Could you check a few things on this model? Use its own coordinates, in mm. Face numbers are marked on the shaded views. A direction names the side the tool comes from. Give positions to 0.01 mm unless a question says otherwise; leave off trailing zeros. Order: outer loops, then holes, each group sorted by start corner. A loop starts at its lowest first (then second) coordinate and runs counter-clockwise, first axis right, second up. Notation, with made-up numbers: M 14.25,75 L 65.25,75 A15 ccw 65.25,80 Z; hole C -37,50 d4. An arc over 180 degrees is marked long. Use a Markdown table: item, result. Add a question column.
Autodesk Inventor part; units mm, degrees
ref_plane "YZ Plane" through (0, 0, 0) normal (1, 0, 0) x (0, 1, 0)
ref_plane "XZ Plane" through (0, 0, 0) normal (0, 1, 0) x (-1, 0, 0)
ref_plane "XY Plane" through (0, 0, 0) normal (0, 0, 1) x (1, 0, 0)
sketch "Sketch1" plane through (0, 0, 0) normal (0, 1, 0) x (-1, 0, 0)
  line L0 (0, 0) -> (-12.7, 0)
  line L1 (-12.7, 0) -> (-12.7, -1.5875)
  line L2 (-12.7, -1.5875) -> (0, -1.5875)
  line L3 (0, -1.5875) -> (0, 0)
  line L4 (0, 0) -> (-4.318, 0)
  line L5 (-4.318, 0) -> (-4.318, -12.7)
  line L6 (-4.318, -12.7) -> (0, -12.7)
  line L7 (0, -12.7) -> (0, 0)
  dimension "d0" = 4.318
  dimension "d1" = 12.7
  dimension "d2" = 12.7
  dimension "d33" = 1.5875
extrude "Extrusion1" add sketch "Sketch1" along normal blind 50.8
sketch "Sketch2" plane through (0, 50.8, 0) normal (0, 1, 0) x (1, 0, 0)
  line L0 (12.7, 0) -> (12.7, 1.5875)
  line L1 (12.7, 1.5875) -> (-4.064, 1.5875)
  line L2 (-4.064, 1.5875) -> (-4.064, -8.5725)
  line L3 (-4.064, -8.5725) -> (12.7, -8.5725)
  line L4 (12.7, -8.5725) -> (12.7, 1.5875)
  line L5 (4.318, 12.7) -> (-4.064, 12.7)
  line L6 (-4.064, 12.7) -> (-4.064, -8.5725)
  line L7 (-4.064, -8.5725) -> (4.318, -8.5725)
  line L8 (4.318, -8.5725) -> (4.318, 12.7)
  dimension "d26" = 10.16
  dimension "d28" = 16.764
extrude "Extrusion2" add sketch "Sketch2" along normal blind 6.35
sketch "Sketch5" plane through (0, 50.8, 0) normal (0, -1, 0) x (1, 0, 0)
  line L0 (12.7, 8.5725) -> (12.7, 0)
  line L1 (-4.064, -12.7) -> (-4.064, 8.5725)
  line L2 (12.7, 8.5725) -> (-4.064, 8.5725)
  line L3 (-4.064, 8.5725) -> (-4.064, 2.1082)
  line L4 (-4.064, 2.1082) -> (12.7, 2.1082)
  line L5 (12.7, 2.1082) -> (12.7, 8.5725)
  line L6 (0, -12.7) -> (-4.064, -12.7)
  line L7 (-4.064, 8.5725) -> (-2.1082, 8.5725)
  line L8 (-2.1082, 8.5725) -> (-2.1082, -12.7)
  line L9 (-2.1082, -12.7) -> (-4.064, -12.7)
  line L10 (-4.064, -12.7) -> (-4.064, 8.5725)
  line L11 (0, -12.7) -> (0, 0)
  line L12 (0, 0) -> (12.7, 0)
  dimension "d29" = 2.1082
  dimension "d30" = 2.1082
extrude "Extrusion4" add sketch "Sketch5" along normal blind 12.7 contours L0 L4 L8 L2 | L8 L4 L1 L2 | L8 L6 L1 L4
sketch "Sketch7" plane through (-4.064, 57.15, -12.7) normal (-1, 0, 0) x (0, 0, 1)
  line L0 (11.1125, 0) -> (11.1125, -57.15)
  line L1 (0, -57.15) -> (0, 0)
  line L2 (11.1125, 0) -> (0, 0)
  line L3 (0, -19.05) -> (14.8082, -19.05)
  line L4 (0, -6.35) -> (12.7, -6.35)
  point P0 (12.7, -57.15)
  point P1 (5.5562, -12.7)
  dimension "d47" = 11.1125
  dimension "d49" = 5.5563
  dimension "d58" = 12.7
  dimension "d59" = 6.35
hole "Hole2" at (-4.064, 44.45, -7.1438) direction (1, 0, 0) diameter 5.1562 depth 1.5875 tip angle 118
sketch "Sketch8" plane through (-4.064, 57.15, -12.7) normal (-1, 0, 0) x (0, 0, 1)
  circle A0 centre (5.5562, -12.7) radius 2.5781
  circle A1 centre (5.5562, -12.7) radius 2.5781
  line L0 (21.2725, 0) -> (21.2725, -19.05)
  line L1 (0, 0) -> (21.2725, 0)
  line L2 (0, -19.05) -> (0, 0)
  line L3 (21.2725, -19.05) -> (0, -19.05)
  point P0 (12.7, -57.15)
extrude "Extrusion5" add sketch "Sketch8" along normal blind 2.413
sketch "Sketch9" plane through (-2.1082, 50.8, 2.1082) normal (1, 0, 0) x (0, 0, -1)
  circle A0 centre (9.2519, -6.35) radius 2.5781
  line L0 (14.8082, -12.7) -> (-6.4643, -12.7)
  line L1 (6.6738, -6.35) -> (11.83, -6.35)
  line L2 (11.83, -6.35) -> (11.83, -12.7)
  line L3 (11.83, -12.7) -> (6.6738, -12.7)
  line L4 (6.6738, -12.7) -> (6.6738, -6.35)
  point P0 (2.1082, -50.8)
  dimension "d62" = 5.1562
extrude "Extrusion6" cut sketch "Sketch9" against normal blind 1.5875
equation "\"d29\" = d30"
properties part number "8GrootTelescope"
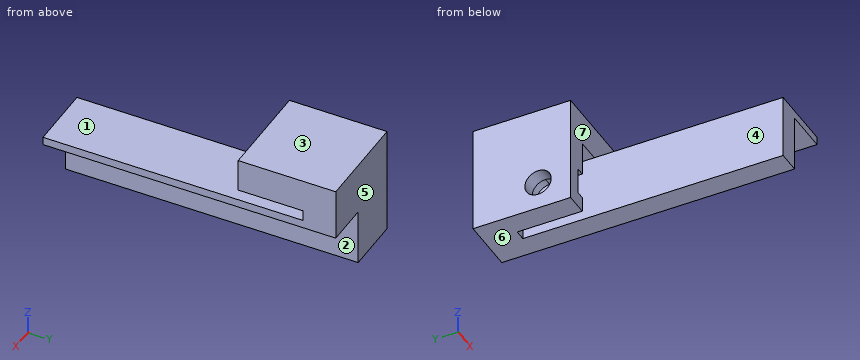
1) For the marked faces 1, 2, 3 and 4, which set-ups out of +Z, -Z, +X, -X, +Y, -Y let a thin tool reach every point of the face, with its end or its side?
2) We'd pull the mould along Y, two halves only. Please class the marked faces 5, 6 and 7: pulls with the +Y half, pulls with the -Y half, needs draft (parallel to the pull), parting line crosses it, or undercut.
3) Suppose I cut it at C-C on y = 37.5. Please give me the cut outline in (x, z).
4) Please list where these lines run through material, in increasing order: line 1 (Z direction, x = 5.75, y = 41); line 2 (Z direction, x = -3.55, y = 44.45); line 3 (Y direction, x = 10.25, z = 0.5). Write a range as from..to.
5) Suppose I cut it at B-B on z = -0.75. Please give me the cut outline in (x, y), and give its area (3 significant figures).
6) Suppose I cut it at A-A on x = 9.5. Please give me the cut outline in (y, z), and give its area (3 significant figures).
7) Suppose I cut it at D-D on z = 1.5. Please give me the cut outline in (x, y).
8) For pin 1 (1.5 mm diameter, centred on x = 5.5, y = 33, fed in from -Z); pin 2 (6.5 mm diameter, centred on y = 30.5, z = -5, fed in from -X); pin 3 (6 mm diameter, centred on y = 44.45, z = -7.14, fed in from +X), each with a flat end and sliding along its axis, tell me the tip position at first contact or that it passes through.
Values found:
| question | item | result |
|---|---|---|
| 1 | face 1 | +X, -Y |
| 1 | face 2 | -Z, +X, +Y, -Y |
| 1 | face 3 | +Z, +X, -X, +Y, -Y |
| 1 | face 4 | -Z, -Y |
| 2 | face 5 | pulls with the +Y half |
| 2 | face 6 | needs draft |
| 2 | face 7 | pulls with the -Y half |
| 3 | outline | M 0,-12.7 L 4.32,-12.7 L 4.32,-1.59 L 12.7,-1.59 L 12.7,0 L 0,0 Z |
| 4 | line 1 | z = -1.59..0, 2.11..8.57 |
| 4 | line 2 | z = -12.7..-9.72, -4.57..8.57 |
| 4 | line 3 | y = 50.8..57.15 |
| 5 | outline | M -6.48,38.1 L -2.11,38.1 L -2.11,50.8 L 0,50.8 L 0,0 L 12.7,0 L 12.7,57.15 L -6.48,57.15 Z |
| 5 | area | 822 mm^2 |
| 6 | outline | M 0,-1.59 L 57.15,-1.59 L 57.15,8.57 L 38.1,8.57 L 38.1,2.11 L 50.8,2.11 L 50.8,0 L 0,0 Z |
| 6 | area | 227 mm^2 |
| 7 | outline | M -6.48,38.1 L -2.11,38.1 L -2.11,50.8 L 12.7,50.8 L 12.7,57.15 L -6.48,57.15 Z |
| 8 | pin 1 | stops at z = -1.59 |
| 8 | pin 2 | stops at x = 0 |
| 8 | pin 3 | stops at x = 4.32 |
